Source: CAD feature listing. Evaluate the final solid. Frame: model axes, mm. A direction names the side the tool comes from. Give positions to 0.01 mm unless a question says otherwise; leave off trailing zeros. Order: outer loops, then holes, each group sorted by start corner. A loop starts at its lowest first (then second) coordinate and runs counter-clockwise, first axis right, second up.
1) Section D-D, the plane y = -2.5. Return loops of the section in (x, z).
2) Draft query along Z for faces 6 (the face through (-25.894, 19.442, -51.907)), 7 (the face through (-91.44, 6.43, -43.2)), 8 (the face through (-83, 22.4, -29)), 9 (the face through (-136.5, 16.57, -84.36)). Return one class per face: released by +Z, released by -Z, zero draft, split by the parting line, or undercut.
3) First-contact query: P1, Ø7.5, axis at x = -67.5, z = 10.5, coming from the -Y side; P2, Ø9.5, axis at x = -82.3, z = 14.1, coming from the +Y side; P3, Ø1, axis at y = 17, z = -49.5, coming from the -X side; P4, Ø3, axis at x = -140, y = 3.5, coming from the -Z side. Flat tips, straight axial feed; report the tip coordinate or a pass-through.
4) Section C-C, the plane x = -153.5. Return loops of the section in (y, z).
5) Section A-A, the plane x = -82.3. Return loops of the section in (y, z), plus the area to 3 significant figures.
6) Material intervals for line 1 (X direction, y = 18, z = -42.8); line 2 (Z direction, x = -82.3, y = 16); line 3 (X direction, y = -1.5, z = -42.8), sorted ascending.
7) Section B-B, the plane z = -42.8. Return loops of the section in (x, y).
8) Access query for faces 1 (the face through (-81.444, -4.93, -14.863)), 2 (the face through (-11, 10.9, -42)), 3 (the face through (-32, -6.4, -43)), 4 (the face through (-81, 6, -85.6)), 5 (the face through (-83, 10.9, 7)). Directions: +Z, -Z, +X, -X, +Y, -Y. A direction counts if a zero-diameter tool reaches every point of the face in a straight line with its end or side. Return the directions, or none.
Autodesk Inventor part; units mm, degrees
ref_plane "YZ Plane" through (0, 0, 0) normal (1, 0, 0) x (0, 1, 0)
ref_plane "XZ Plane" through (0, 0, 0) normal (0, 1, 0) x (-1, 0, 0)
ref_plane "XY Plane" through (0, 0, 0) normal (0, 0, 1) x (1, 0, 0)
sketch "Sketch1" plane through (0, 0, 0) normal (1, 0, 0) x (0, 1, 0)
  line L0 (0, 0) -> (10.9, 0)
  line L1 (10.9, 0) -> (10.9, -85.6)
  line L2 (10.9, -85.6) -> (0, -85.6)
  line L3 (0, -85.6) -> (0, -66.6)
  line L4 (-10, -74.991) -> (-10, -10.609)
  line L5 (-10, -74.991) -> (0, -66.6)
  line L6 (0, 0) -> (0, -19)
  line L7 (0, -19) -> (-10, -10.609)
  line L8 (0, -66.6) -> (0, -19)
  line L9 (0, -42.8) -> (-10, -42.8) construction
  dimension "d1" = 85.6
  dimension "d7" = 19
  dimension "d30" = 50
  dimension "d31" = 19
  dimension "d32" = 50
  dimension "d33" = 10
extrude "Extrusion1" add sketch "Sketch1" against normal blind 165.2
sketch "Sketch2" plane through (0, 10.9, 0) normal (0, 1, 0) x (1, 0, 0)
  point P0 (0, 0)
sketch "Sketch3" plane through (0, 10.9, 0) normal (0, 1, 0) x (1, 0, 0)
  line L0 (0, 0) -> (0, 85.6)
  line L1 (0, 42.8) -> (-14, 42.8)
  line L2 (-14, 42.8) -> (-82.3, 42.8)
  circle A0 centre (-82.3, 42.8) radius 68.3
  dimension "d10" = 14
  dimension "d11" = 68.3
extrude "Extrusion2" add sketch "Sketch3" along normal blind 11.5
sketch "Sketch4" plane through (-82.3, 22.4, -42.8) normal (0, 1, 0) x (1, 0, 0)
  circle A0 centre (0, 0) radius 9.15
  point P0 (82.3, -42.8)
  dimension "d14" = 18.3
extrude "Extrusion3" cut sketch "Sketch4" against normal blind 73.75
sketch "Sketch5" plane through (-82.3, 22.4, -42.8) normal (0, 1, 0) x (1, 0, 0)
  circle A0 centre (0, 0) radius 68.3
  line L0 (0, 68.3) -> (0, 62.3)
  line L1 (0, -68.3) -> (0, -62.3)
  line L2 (0, 62.3) -> (0, 56.9)
  circle A1 centre (0, 56.9) radius 5.4
  line L3 (0, -62.3) -> (0, -56.9)
  line L4 (82.3, -32.191) -> (-82.9, -32.191)
  circle A2 centre (0, -56.9) radius 5.4
  point P0 (82.3, -42.8)
  dimension "d17" = 6
  dimension "d18" = 6
  dimension "d19" = 5.4
  dimension "d20" = 5.4
extrude "Extrusion4" cut sketch "Sketch5" against normal blind 73.75 contours A1 | A2
sketch "Sketch6" plane through (-82.3, 22.4, -42.8) normal (0, 1, 0) x (1, 0, 0)
  point P0 (82.3, -42.8)
sketch "Sketch7" plane through (-82.3, 22.4, -42.8) normal (0, 1, 0) x (1, 0, 0)
  circle A0 centre (0, 0) radius 68.3
  line L0 (68.3, 0) -> (61.4, 0)
  line L1 (61.4, 0) -> (50.6, 0)
  circle A1 centre (50.6, 0) radius 10.8
  point P0 (82.3, -42.8)
  dimension "d23" = 6.9
  dimension "d24" = 10.8
extrude "Extrusion5" cut sketch "Sketch7" against normal blind 6 contours A1
sketch "Sketch8" plane through (-31.7, 16.4, -42.8) normal (0, 1, 0) x (1, 0, 0)
  circle A0 centre (0, 0) radius 3.1
  point P0 (31.7, -42.8)
  dimension "d27" = 6.2
extrude "Extrusion6" cut sketch "Sketch8" against normal blind 22.8
ref_plane "Work Plane1" through (0, 0, -42.8) normal (0, 0, -1) x (-1, 0, 0)
properties part number "Top Part Tool bit"
From the geometry:
1. outline: (-165.2, -68.7) - (0, -68.7) - (0, -16.9) - (-165.2, -16.9) - close; hole circle Ø18.3 at (-82.3, -42.8); hole circle Ø6.2 at (-31.7, -42.8)
2. face 6: undercut
2. face 7: undercut
2. face 8: zero draft
2. face 9: split by the parting line
3. P1: stops at y = 10.9
3. P2: passes through
3. P3: stops at x = -150.32
3. P4: stops at z = -85.6
4. outline: (-10, -74.99) - (0, -66.6) - (0, -85.6) - (10.9, -85.6) - (10.9, 0) - (0, 0) - (0, -19) - (-10, -10.61) - close
5. outline: (-10, -74.99) - (0, -66.6) - (0, -85.6) - (10.9, -85.6) - (10.9, -94.3) - (22.4, -94.3) - (22.4, -51.95) - (-10, -51.95) - close; (-10, -33.65) - (22.4, -33.65) - (22.4, 8.7) - (10.9, 8.7) - (10.9, 0) - (0, 0) - (0, -19) - (-10, -10.61) - close; (10.9, -111.1) - (22.4, -111.1) - (22.4, -105.1) - (10.9, -105.1) - close; (10.9, 19.5) - (22.4, 19.5) - (22.4, 25.5) - (10.9, 25.5) - close
5. area: 2,220 mm2
6. line 1: x = -150.6 to -91.45, -73.15 to -42.5, -20.9 to -14
6. line 2: z = -111.1 to -105.1, -94.3 to -51.95, -33.65 to 8.7, 19.5 to 25.5
6. line 3: x = -165.2 to -91.45, -73.15 to -34.8, -28.6 to 0
7. outline: (-165.2, -10) - (-91.45, -10) - (-91.45, 22.4) - (-150.6, 22.4) - (-150.6, 10.9) - (-165.2, 10.9) - close; (-73.15, -10) - (0, -10) - (0, 10.9) - (-14, 10.9) - (-14, 22.4) - (-20.9, 22.4) - (-20.9, 16.4) - (-28.6, 16.4) - (-28.6, -6.4) - (-34.8, -6.4) - (-34.8, 16.4) - (-42.5, 16.4) - (-42.5, 22.4) - (-73.15, 22.4) - close
8. face 1: +Z, +X, -X
8. face 2: +X, +Y
8. face 3: +Y
8. face 4: -Z, +X, -X, -Y
8. face 5: +Z, +X, -X, -Y
